Can you work these out from the model? Positions are in its coordinate system, mm. A direction names the side the tool comes from. Round coordinates to 2 decimals unless told otherwise and drop trailing zeros. Order: outer loops, then holes, each group sorted by start corner. A loop starts at its lowest first (then second) coordinate and runs counter-clockwise, first axis right, second up.
Q1. If we section it at A-A (z = -1): Please give me the cut outline in (x, y).
Q2. If we section it at B-B (y = 19.5): Please give me the cut outline in (x, z), plus the area to 3 significant figures.
Q3. We'd pull the mould along Y, two halves only. Please class faces 5 (the face through (8, -2.5, -15)), 6 (the face through (1.493, 21.037, -16.298)), 7 (the face through (14, -6, 15)): pulls with the +Y half, pulls with the -Y half, needs draft (parallel to the pull), parting line crosses it, or undercut.
Q4. If I drill on line 1 (Z direction, x = 8.2, y = -5.75); line 2 (Y direction, x = 1.45, z = -16.5); line 3 (X direction, y = -15, z = -16), over which ranges is the centre line in solid material (lowest first)?
Q5. If we section it at C-C (x = 13): Please give me the cut outline in (y, z), plus the area to 3 significant figures.
Q6. For faces 1 (the face through (8, -7, 11.5)), 2 (the face through (8, -7, -17.5)), 3 (the face through (0.986, 10.39, 16.107)), 4 (the face through (8, -7, 17.5)), which set-ups out of +Z, -Z, +X, -X, +Y, -Y let a thin tool reach every point of the face, with its end or its side?
Q7. If we section it at D-D (x = 8.2): Please give me the cut outline in (y, z), plus the area to 3 significant figures.
Q8. Will these pins go through, and if not, where does the flat tip stop? P1, Ø5, axis at y = 19.5, z = -16.5, coming from the -X side; P2, Ø4, axis at x = 10, z = -15, coming from the +Y side; P3, Ø5, axis at x = 5, z = -15.5, coming from the -Y side; P4, Ø1.4, axis at x = 8.2, z = 13.75, coming from the -Y side.
from build123d import *
from OCP.BRepFilletAPI import BRepFilletAPI_MakeChamfer

# Parameters (mm, degrees)
SKETCH1_W               = 39
SKETCH1_H               = 45
SKETCH1_R               = 1.55
BOSS_EXTRUDE1_DEPTH     = 2
SKETCH2_W               = 6
SKETCH2_H               = 7
BOSS_EXTRUDE2_DEPTH     = 12
CHAMFER1_SIZE           = 5
CHAMFER1_SIZE_2         = 12
CUT_EXTRUDE1_DEPTH      = 12
CUT_EXTRUDE1_DEPTH_BACK = 22
SKETCH3_R               = 0.75
CUT_EXTRUDE2_DEPTH      = 33.101401839
CUT_EXTRUDE2_DEPTH_BACK = 33.101401839
SKETCH4_W               = 39
SKETCH4_H               = 45
SKETCH4_W_2             = 38.7
SKETCH4_H_2             = 44.7
FILLET1_R               = 1
CHAMFER2_SIZE           = 1


with BuildPart() as part:
    # Sketch1 → Boss-Extrude1 (new body)
    with BuildSketch(Plane(origin=(0, 0, 0), x_dir=(0, 0, -1), z_dir=(1, 0, 0))):
        Rectangle(SKETCH1_W, SKETCH1_H)
        with Locations((-16.5, 19.5)):
            Circle(SKETCH1_R, mode=Mode.SUBTRACT)
        with Locations((16.5, 19.5)):
            Circle(SKETCH1_R, mode=Mode.SUBTRACT)
        with Locations((16.5, -19.5)):
            Circle(SKETCH1_R, mode=Mode.SUBTRACT)
        with Locations((-16.5, -19.5)):
            Circle(SKETCH1_R, mode=Mode.SUBTRACT)
        with BuildLine():
            Line((-11.118955155, 15.489657916), (11.118955155, 15.489657916))
            ThreePointArc((11.118955155, 15.489657916), (16.108613071, 10.5), (11.118955155, 5.510342084))
            Line((11.118955155, 5.510342084), (-11.118955155, 5.510342084))
            ThreePointArc((-11.118955155, 5.510342084), (-16.108613071, 10.5), (-11.118955155, 15.489657916))
        make_face(mode=Mode.SUBTRACT)
    extrude(amount=BOSS_EXTRUDE1_DEPTH)

    # Sketch2 → Boss-Extrude2 (add)
    with BuildSketch(Plane(origin=(2, 0, 0), x_dir=(0, 0, -1), z_dir=(1, 0, 0))):
        with Locations((14.5, -6)):
            Rectangle(SKETCH2_W, SKETCH2_H)
        with Locations((-14.5, -6)):
            Rectangle(SKETCH2_W, SKETCH2_H)
    extrude(amount=BOSS_EXTRUDE2_DEPTH)

    # Chamfer1
    chamfer1_edges_1 = [part.edges().sort_by_distance(p)[0] for p in [
        (2, -9.5, -14.5),
    ]]
    chamfer1_side_1 = [part.faces().sort_by_distance(p)[0] for p in [
        (2, -9.6, -14.5),
    ]]
    chamfer1_edges_2 = [part.edges().sort_by_distance(p)[0] for p in [
        (2, -9.5, 14.5),
    ]]
    chamfer1_side_2 = [part.faces().sort_by_distance(p)[0] for p in [
        (2, -9.6, 14.5),
    ]]
    chamfer1 = BRepFilletAPI_MakeChamfer(part.part.solid().wrapped)
    for e in chamfer1_edges_1:
        chamfer1.Add(CHAMFER1_SIZE - 0.0001, CHAMFER1_SIZE_2 - 0.0001, e.wrapped, chamfer1_side_1[0].wrapped)
    for e in chamfer1_edges_2:
        chamfer1.Add(CHAMFER1_SIZE - 0.0001, CHAMFER1_SIZE_2 - 0.0001, e.wrapped, chamfer1_side_2[0].wrapped)
    add(Compound.cast(chamfer1.Shape()), mode=Mode.REPLACE)  # a hair under: the kernel refuses the full size

    # Sketch3 → Cut-Extrude1 (cut, two sides: drawn at the far end of the back side and taken through both)
    with BuildSketch(Plane(origin=(0, -2.5, 0), x_dir=(1, 0, 0), z_dir=(0, 1, 0)).offset(-CUT_EXTRUDE1_DEPTH_BACK)):
        with Locations(Location((8.2, -13.75, 0), (0, 0, 90))):
            Circle(SKETCH3_R)
        with Locations(Location((8.2, 13.75, 0), (0, 0, 90))):
            Circle(SKETCH3_R)
    extrude(amount=CUT_EXTRUDE1_DEPTH + CUT_EXTRUDE1_DEPTH_BACK, mode=Mode.SUBTRACT)

    # Sketch4 → Cut-Extrude2 (cut, two sides: drawn at the far end of the back side and taken through both)
    with BuildSketch(Plane(origin=(2, 0, 0), x_dir=(0, 0, -1), z_dir=(1, 0, 0)).offset(-CUT_EXTRUDE2_DEPTH_BACK)):
        Rectangle(SKETCH4_W, SKETCH4_H)
        Rectangle(SKETCH4_W_2, SKETCH4_H_2, mode=Mode.SUBTRACT)
    extrude(amount=CUT_EXTRUDE2_DEPTH + CUT_EXTRUDE2_DEPTH_BACK, mode=Mode.SUBTRACT)

    # Fillet1
    fillet1_edges = [part.edges().sort_by_distance(p)[0] for p in [
        (1, 22.35, -19.35),
        (1, -22.35, -19.35),
        (1, -22.35, 19.35),
        (1, 22.35, 19.35),
    ]]
    fillet(fillet1_edges, radius=FILLET1_R)

    # Chamfer2
    chamfer2_edges = [part.edges().sort_by_distance(p)[0] for p in [
        (0, 19.5, 18.05),
        (0, 19.5, -14.95),
        (0, -19.5, -14.95),
        (0, -19.5, 18.05),
    ]]
    chamfer(chamfer2_edges, length=CHAMFER2_SIZE)


solid = part.part
Solution:
1. outline: (0, -22.35) - (2, -22.35) - (2, 5.51) - (0, 5.51) - close; (0, 15.49) - (2, 15.49) - (2, 22.35) - (0, 22.35) - close
2. outline: (0, -19.35) - (2, -19.35) - (2, -18.05) - (1, -18.05) - (0, -19.05) - close; (0, -13.95) - (1, -14.95) - (2, -14.95) - (2, 14.95) - (1, 14.95) - (0, 13.95) - close; (0, 19.05) - (1, 18.05) - (2, 18.05) - (2, 19.35) - (0, 19.35) - close
2. area: 63.0 mm2
3. face 5: pulls with the +Y half
3. face 6: undercut
3. face 7: needs draft
4. line 1: z = -17.5 to -14.5, -13 to -11.5, 11.5 to 13, 14.5 to 17.5
4. line 2: y = -22.35 to -21.05, -17.95 to 17.95, 21.05 to 22.35
4. line 3: x = 0 to 2
5. outline: (-9.92, -17.5) - (-2.5, -17.5) - (-2.5, -11.5) - (-9.92, -11.5) - close; (-9.92, 11.5) - (-2.5, 11.5) - (-2.5, 17.5) - (-9.92, 17.5) - close
5. area: 89.0 mm2
6. face 1: +X, +Y, -Y
6. face 2: -Z, +X, +Y, -Y
6. face 3: +X, -X
6. face 4: +Z, +X, +Y, -Y
7. outline: (-11.92, -17.5) - (-2.5, -17.5) - (-2.5, -14.5) - (-11.92, -14.5) - close; (-11.92, -13) - (-2.5, -13) - (-2.5, -11.5) - (-11.92, -11.5) - close; (-11.92, 11.5) - (-2.5, 11.5) - (-2.5, 13) - (-11.92, 13) - close; (-11.92, 14.5) - (-2.5, 14.5) - (-2.5, 17.5) - (-11.92, 17.5) - close
7. area: 84.7 mm2
8. P1: stops at x = 0.05
8. P2: stops at y = -2.5
8. P3: stops at y = -14.29
8. P4: passes through
